Work out the finished part from the listing and answer in its coordinate system (mm). Give positions to 0.01 mm unless a question says otherwise; leave off trailing zeros. Order: outer loops, then holes, each group sorted by start corner. A loop starts at its lowest first (then second) coordinate and runs counter-clockwise, first axis right, second up. Notation, with made-up numbers: (-23, 57) - (-2, 57) arc R20 cw to (-2, 73) - close; hole circle Ø6 at (-15.5, 61.5). An arc over 180 degrees is marked (long way). Return JSON: item names as keys, results as strings. Group by question number.
Autodesk Inventor part; units mm, degrees
ref_plane "YZ Plane" through (0, 0, 0) normal (1, 0, 0) x (0, 1, 0)
ref_plane "XZ Plane" through (0, 0, 0) normal (0, 1, 0) x (-1, 0, 0)
ref_plane "XY Plane" through (0, 0, 0) normal (0, 0, 1) x (1, 0, 0)
sketch "Sketch1" plane through (0, 0, 0) normal (0, 1, 0) x (-1, 0, 0)
  line L0 (-25.4, 25.4) -> (25.4, 25.4)
  line L1 (25.4, 25.4) -> (25.4, -25.4)
  line L2 (25.4, -25.4) -> (-25.4, -25.4)
  line L3 (-25.4, -25.4) -> (-25.4, 25.4)
  line L4 (-25.4, 25.4) -> (25.4, -25.4) construction
  line L5 (25.4, 25.4) -> (-25.4, -25.4) construction
  point P0 (0, 0)
  dimension "d0" = 50.8
  dimension "d1" = 50.8
extrude "Extrusion1" add sketch "Sketch1" along normal blind 2.9718
sketch "Sketch2" plane through (0, 2.9718, 0) normal (0, 1, 0) x (1, 0, 0)
  line L0 (-25.4, -25.4) -> (25.4, -25.4)
  line L1 (-25.4, -25.4) -> (-22.4282, -25.4)
  line L2 (-22.4282, -25.4) -> (-22.4282, -12.7)
  line L3 (-22.4282, -12.7) -> (-25.4, -12.7)
  line L4 (-25.4, -12.7) -> (-25.4, -25.4)
  line L5 (-25.4, 25.4) -> (-25.4, -25.4)
  line L6 (-25.4, 0) -> (-22.4282, 0)
  line L7 (-22.4282, 0) -> (-22.4282, 12.7)
  line L8 (-22.4282, 12.7) -> (-25.4, 12.7)
  line L9 (-25.4, 12.7) -> (-25.4, 0)
  line L10 (-25.4, 25.4) -> (-12.7, 25.4)
  line L11 (-12.7, 25.4) -> (-12.7, 22.4282)
  line L12 (-12.7, 22.4282) -> (-25.4, 22.4282)
  line L13 (-25.4, 22.4282) -> (-25.4, 25.4)
  line L14 (25.4, 25.4) -> (-25.4, 25.4)
  line L15 (0, 25.4) -> (12.7, 25.4)
  line L16 (12.7, 25.4) -> (12.7, 22.4282)
  line L17 (12.7, 22.4282) -> (0, 22.4282)
  line L18 (0, 22.4282) -> (0, 25.4)
  point P0 (0, 0)
  dimension "d4" = 2.9718
  dimension "d5" = 12.7
  dimension "d6" = 2.9718
  dimension "d7" = 12.7
  dimension "d8" = 12.7
  dimension "d9" = 2.9718
  dimension "d10" = 12.7
  dimension "d11" = 2.9718
extrude "Extrusion2" cut sketch "Sketch2" against normal blind 2.9718
sketch "Sketch3" plane through (0, 0, 0) normal (0, -1, 0) x (1, 0, 0)
  line L0 (7.7851, -12.7) -> (4.9149, -12.7)
  line L1 (4.9149, -22.4282) -> (7.7851, -22.4282)
  line L2 (7.7851, -12.7) -> (4.9149, -22.4282) construction
  line L3 (4.9149, -12.7) -> (7.7851, -22.4282) construction
  line L4 (0, -22.4282) -> (12.7, -22.4282)
  line L5 (12.7, -22.4282) -> (12.7, -25.4)
  line L6 (2.6797, -14.0462) -> (2.6797, -16.5862)
  line L7 (10.0203, -16.5862) -> (10.0203, -14.0462)
  line L8 (10.0203, -14.0462) -> (2.6797, -16.5862) construction
  line L9 (2.6797, -14.0462) -> (10.0203, -16.5862) construction
  line L10 (2.6797, -16.5862) -> (4.9149, -16.5862)
  line L11 (4.9149, -12.7) -> (4.9149, -14.0462)
  line L12 (4.9149, -16.5862) -> (4.9149, -22.4282)
  line L13 (10.0203, -14.0462) -> (7.7851, -14.0462)
  line L14 (4.9149, -14.0462) -> (2.6797, -14.0462)
  line L15 (7.7851, -22.4282) -> (7.7851, -16.5862)
  line L16 (7.7851, -14.0462) -> (7.7851, -12.7)
  line L17 (7.7851, -16.5862) -> (10.0203, -16.5862)
  line L18 (-14.0462, -10.0203) -> (-16.5862, -10.0203)
  line L19 (-16.5862, -10.0203) -> (-16.5862, -7.7851)
  line L20 (-16.5862, -7.7851) -> (-22.4282, -7.7851)
  line L21 (-22.4282, -7.7851) -> (-22.4282, -4.9149)
  line L22 (-22.4282, -4.9149) -> (-16.5862, -4.9149)
  line L23 (-16.5862, -4.9149) -> (-16.5862, -2.6797)
  line L24 (-16.5862, -2.6797) -> (-14.0462, -2.6797)
  line L25 (-14.0462, -2.6797) -> (-14.0462, -4.9149)
  line L26 (-14.0462, -4.9149) -> (-12.7, -4.9149)
  line L27 (-12.7, -4.9149) -> (-12.7, -7.7851)
  line L28 (-12.7, -7.7851) -> (-14.0462, -7.7851)
  line L29 (-14.0462, -7.7851) -> (-14.0462, -10.0203)
  line L30 (-25.4, 0) -> (-22.4282, 0)
  line L31 (-22.4282, -12.7) -> (-22.4282, 0)
  line L32 (-14.0462, 17.6149) -> (-14.0462, 15.3797)
  line L33 (-12.7, 17.6149) -> (-14.0462, 17.6149)
  line L34 (-12.7, 20.4851) -> (-12.7, 17.6149)
  line L35 (-14.0462, 15.3797) -> (-16.5862, 15.3797)
  line L36 (-14.0462, 20.4851) -> (-12.7, 20.4851)
  line L37 (-14.0462, 22.7203) -> (-14.0462, 20.4851)
  line L38 (-16.5862, 22.7203) -> (-14.0462, 22.7203)
  line L39 (-16.5862, 15.3797) -> (-16.5862, 17.6149)
  line L40 (-16.5862, 20.4851) -> (-16.5862, 22.7203)
  line L41 (-22.4282, 20.4851) -> (-16.5862, 20.4851)
  line L42 (-16.5862, 17.6149) -> (-22.4282, 17.6149)
  line L43 (-22.4282, 17.6149) -> (-22.4282, 20.4851)
  point P0 (0, 0)
  point P1 (6.35, -17.5641)
  point P2 (6.35, -15.3162)
  dimension "d14" = 0
  dimension "d15" = 2.8702
  dimension "d16" = 6.35
  dimension "d17" = 9.7282
  dimension "d18" = 7.3406
  dimension "d19" = 0
  dimension "d20" = 2.54
  dimension "d22" = 5.842
  dimension "d23" = 2.2352
  dimension "d24" = 5.842
  dimension "d25" = 2.8702
  dimension "d26" = 1.3462
  dimension "d46" = 2.8702
  dimension "d47" = 5.842
  dimension "d48" = 2.2352
  dimension "d49" = 2.2352
  dimension "d50" = 1.3462
  dimension "d51" = 2.54
  dimension "d52" = 2.54
  dimension "d60" = 4.9149
  dimension "d61" = 0
  dimension "d64" = 25.4
extrude "Extrusion4" cut sketch "Sketch3" against normal blind 25.4
properties part number "base"
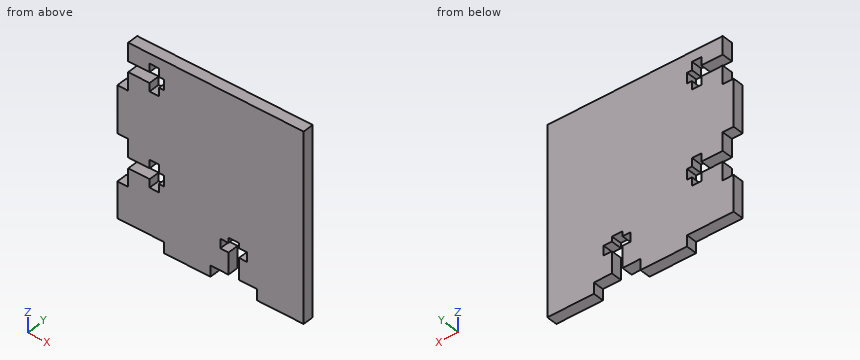
1. The part is cut by section C-C (z = 18.5). Give the vertices of the cut face in (x, y), and give its area (3 significant figures).
2. Consider probe 1 along Z at (x, y) = (-17, 0.55); probe 2 along X at (y, z) = (1.2, 22); probe 3 along X at (y, z) = (1.25, -20.5). Determine where each line is inside the solid, lowest interval first. Write a range as from..to.
3. The part is cut by section A-A (x = 8.5). Give the vertices of the cut face in (y, z).
4. The part is cut by section B-B (z = -19.5). Give the vertices of the cut face in (x, y).
5. Each of these flat-tipped pins is pushed along its axis until it touches: pin 1 (1.4 mm diameter, centred on y = 2, z = 18.5, fed in from -X); pin 2 (0.9 mm diameter, centred on x = -19, y = 1.5, fed in from -Z). Where does it stop, or does it pass through?
Answers:
{
 "1": {"outline": "(-12.7, 0) - (25.4, 0) - (25.4, 2.97) - (-12.7, 2.97) - close", "area": "113 mm^2"},
 "2": {"probe 1": "z = -22.43..-7.79, -4.91..17.61, 20.49..25.4", "probe 2": "x = -22.43..-16.59, -14.05..25.4", "probe 3": "x = -25.4..4.91, 7.79..25.4"},
 "3": {"outline": "(0, -22.43) - (2.97, -22.43) - (2.97, -16.59) - (0, -16.59) - close; (0, -14.05) - (2.97, -14.05) - (2.97, 25.4) - (0, 25.4) - close"},
 "4": {"outline": "(-25.4, 0) - (4.91, 0) - (4.91, 2.97) - (-25.4, 2.97) - close; (7.79, 0) - (25.4, 0) - (25.4, 2.97) - (7.79, 2.97) - close"},
 "5": {"pin 1": "stops at x = -12.7", "pin 2": "stops at z = -22.43"}
}
